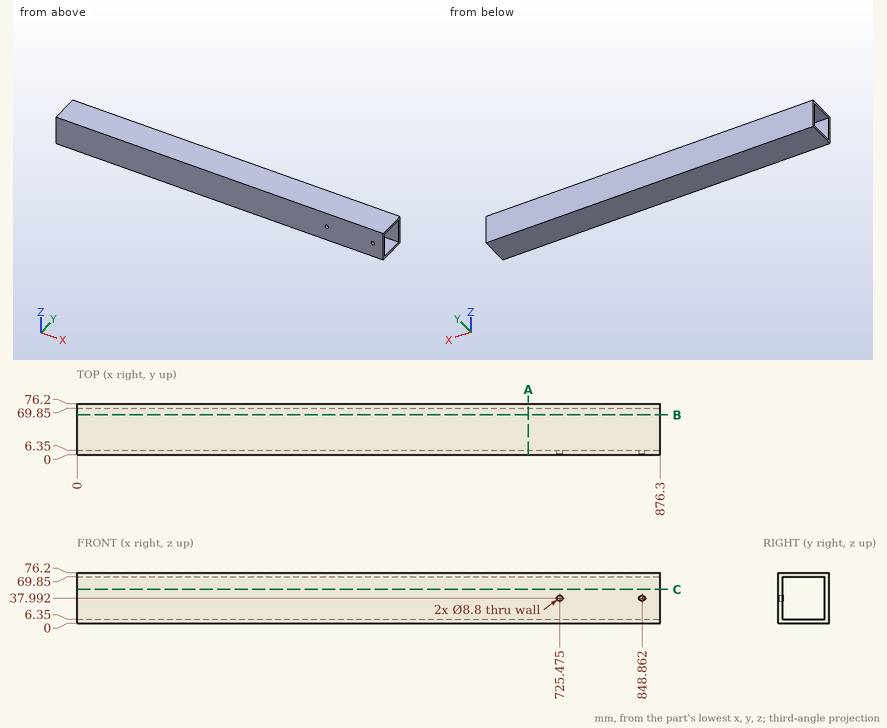
Study the drawing (mm; zero at the part's minimum x, y, z) and answer. Coordinates: 2 decimals unless noted, no trailing zeros. Loops run counter-clockwise (first coordinate to the right, second up) from the corner with the lowest first, then second, coordinate; pieces in that order, holes last. Notation, with made-up numbers: (-17.75, -14) -> (9.25, -14) arc R13 cw to (9.25, -7) -> close; hole circle Ø6 at (-5.75, 82). An arc over 180 degrees is marked (long way). Write item = value, one per line. Start each with the question number.
1) Find the intervals of material crossed by L1, parallel to Y at x = 543, z = 14, in increasing order. Write a range as from..to.
2) Given P1, Ø10, axis at x = 369.5, y = 41, coming from the -Z side; P2, Ø8, axis at y = 26.5, z = 11, coming from the -X side, each flat-ended and moving along its own axis, determine where each tip first touches the part or whether it passes through.
3) The part is cut by section B-B, the plane y = 60. Determine the outline of the cut face in (x, z), plus the area to 3 significant figures.
4) The part is cut by section A-A, the plane x = 678. Determine the outline of the cut face in (y, z).
Result:
q1.L1 = 0..6.35, 69.85..76.2
q2.P1 = 0
q2.P2 = through
q3.outline = (0, 0) -> (876.3, 0) -> (876.3, 6.35) -> (0, 6.35) -> close; (0, 69.85) -> (876.3, 69.85) -> (876.3, 76.2) -> (0, 76.2) -> close
q3.area = 11,100 mm²
q4.outline = (0, 0) -> (76.2, 0) -> (76.2, 76.2) -> (0, 76.2) -> close; hole (6.35, 6.35) -> (69.85, 6.35) -> (69.85, 69.85) -> (6.35, 69.85) -> close
